Work out the finished part from the listing and answer in its coordinate system (mm). Face numbers are marked on the shaded views. A direction names the side the tool comes from. Round coordinates to 2 decimals unless told otherwise and drop trailing zeros. Write each loop counter-clockwise with the first axis right and the second up, starting at its lowest first coordinate (ties: lowest second). Pieces come first, ordered by that corner, then holes. Notation, with made-up numbers: M -4.5,-6.75 L -0.5,-6.75 A20 ccw -0.5,0.25 Z; hole C -4,74.25 d9. An arc over 180 degrees is marked long. Answer in a Markdown table with one row per item.
```python
from build123d import *

# Parameters (mm, degrees)
SKETCH_1_W          = 15
SKETCH_1_H          = 15
SKETCH_1_W_2        = 12
SKETCH_1_H_2        = 12
EXTRUDE_2_DEPTH     = 85
SKETCH_3_R          = 1.5
CUT_EXTRUDE_2_DEPTH = 10
SKETCH_4_R          = 1.5
CUT_EXTRUDE_3_DEPTH = 10
SKETCH_5_R          = 4
CUT_EXTRUDE_4_DEPTH = 10
SKETCH_6_R          = 4
CUT_EXTRUDE_5_DEPTH = 10
SKETCH_7_R          = 3
CUT_EXTRUDE_6_DEPTH = 10
SKETCH_8_R          = 1.5
CUT_EXTRUDE_7_DEPTH = 10
SKETCH_9_R          = 1.5
CUT_EXTRUDE_8_DEPTH = 10
SKETCH_10_R         = 4
CUT_EXTRUDE_9_DEPTH = 10


with BuildPart() as part:
    # ｽｹｯﾁ1 → ﾎﾞｽ - 押し出し2 (new body)
    with BuildSketch(Plane.XY):
        with Locations((0.489915859, 0.232626086)):
            Rectangle(SKETCH_1_W, SKETCH_1_H)
        with Locations((0.489915859, 0.232626086)):
            Rectangle(SKETCH_1_W_2, SKETCH_1_H_2, mode=Mode.SUBTRACT)
    extrude(amount=EXTRUDE_2_DEPTH)

    # ｽｹｯﾁ3 → ｶｯﾄ - 押し出し2 (cut)
    with BuildSketch(Plane(origin=(0, 7.732626086, 0), x_dir=(1, 0, 0), z_dir=(0, 1, 0))):
        with Locations((0.489915859, -77.5)):
            Circle(SKETCH_3_R)
    extrude(amount=-CUT_EXTRUDE_2_DEPTH, mode=Mode.SUBTRACT)

    # ｽｹｯﾁ4 → ｶｯﾄ - 押し出し3 (cut)
    with BuildSketch(Plane(origin=(7.989915859, 0, 0), x_dir=(0, 0, -1), z_dir=(1, 0, 0))):
        with Locations((-62.5, 0.232626086)):
            Circle(SKETCH_4_R)
    extrude(amount=-CUT_EXTRUDE_3_DEPTH, mode=Mode.SUBTRACT)

    # ｽｹｯﾁ5 → ｶｯﾄ - 押し出し4 (cut)
    with BuildSketch(Plane.XZ.offset(7.267373914)):
        with Locations((0.489915859, 77.5)):
            Circle(SKETCH_5_R)
    extrude(amount=-CUT_EXTRUDE_4_DEPTH, mode=Mode.SUBTRACT)

    # ｽｹｯﾁ6 → ｶｯﾄ - 押し出し5 (cut)
    with BuildSketch(Plane.ZY.offset(7.010084141)):
        with Locations((62.5, 0.232626086)):
            Circle(SKETCH_6_R)
    extrude(amount=-CUT_EXTRUDE_5_DEPTH, mode=Mode.SUBTRACT)

    # ｽｹｯﾁ7 → ｶｯﾄ - 押し出し6 (cut)
    with BuildSketch(Plane.ZY.offset(7.010084141)):
        with Locations((16, 0.232626086)):
            Circle(SKETCH_7_R)
    extrude(amount=-CUT_EXTRUDE_6_DEPTH, mode=Mode.SUBTRACT)

    # ｽｹｯﾁ8 → ｶｯﾄ - 押し出し7 (cut)
    with BuildSketch(Plane.ZY.offset(7.010084141)):
        with Locations((5, 0.232626086)):
            Circle(SKETCH_8_R)
    extrude(amount=-CUT_EXTRUDE_7_DEPTH, mode=Mode.SUBTRACT)

    # ｽｹｯﾁ9 → ｶｯﾄ - 押し出し8 (cut)
    with BuildSketch(Plane.ZY.offset(7.010084141)):
        with Locations((27, 0.232626086)):
            Circle(SKETCH_9_R)
    extrude(amount=-CUT_EXTRUDE_8_DEPTH, mode=Mode.SUBTRACT)

    # ｽｹｯﾁ10 → ｶｯﾄ - 押し出し9 (cut)
    with BuildSketch(Plane(origin=(7.989915859, 0, 0), x_dir=(0, 0, -1), z_dir=(1, 0, 0))):
        with Locations((-16, 0.232626086)):
            Circle(SKETCH_10_R)
        with Locations((-27, 0.232626086)):
            Circle(SKETCH_10_R)
    extrude(amount=-CUT_EXTRUDE_9_DEPTH, mode=Mode.SUBTRACT)


solid = part.part
```
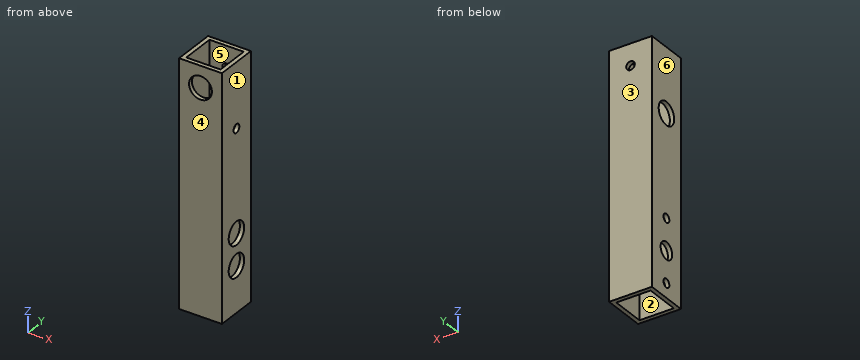
1. Given pin 1 (5 mm diameter, centred on x = 0.49, z = 77.5, fed in from +Y); pin 2 (5 mm diameter, centred on x = 0.49, z = 77.5, fed in from -Y); pin 3 (5 mm diameter, centred on y = 0.23, z = 62.5, fed in from -X), each flat-ended and moving along its own axis, determine where each tip first touches the part or whether it passes through.
Calculated:
| item | result |
|---|---|
| pin 1 | stops at y = 7.73 |
| pin 2 | stops at y = 6.23 |
| pin 3 | stops at x = 6.49 |
2. Determine the mould class of the marked faces 1, 2, 3 and 4 for opening direction Y: released by +Y, released by -Y, zero draft, split by the parting line, or undercut.
Calculated:
| item | result |
|---|---|
| face 1 | zero draft |
| face 2 | undercut |
| face 3 | released by +Y |
| face 4 | released by -Y |
3. The part is cut by section C-C (z = 62). Determine the outline of the cut face in (x, y), plus the area to 3 significant figures.
Calculated:
| item | result |
|---|---|
| outline | M -7.01,-7.27 L 7.99,-7.27 L 7.99,-1.18 L 6.49,-1.18 L 6.49,-5.77 L -5.51,-5.77 L -5.51,-3.74 L -7.01,-3.74 Z; M -7.01,4.2 L -5.51,4.2 L -5.51,6.23 L 6.49,6.23 L 6.49,1.65 L 7.99,1.65 L 7.99,7.73 L -7.01,7.73 Z |
| area | 64.9 mm² |
4. The part is cut by section B-B (y = -4.5). Determine the outline of the cut face in (x, z).
Calculated:
| item | result |
|---|---|
| outline | M -7.01,0 L -5.51,0 L -5.51,85 L -7.01,85 Z; M 6.49,0 L 7.99,0 L 7.99,85 L 6.49,85 Z |
5. Consider line 1 along Y through (x, z) = (5.75, 58); line 2 along X through (y, z) = (7.3, 77.5); line 3 along Y through (x, z) = (-6.25, 5). Determine where each line is inside the solid, lowest interval first. Write a range as from..to.
Calculated:
| item | result |
|---|---|
| line 1 | y = -7.27..-5.77, 6.23..7.73 |
| line 2 | x = -7.01..-1.01, 1.99..7.99 |
| line 3 | y = -7.27..-1.27, 1.73..7.73 |
6. The part is cut by section A-A (z = 39). Determine the outline of the cut face in (x, y), plus the area to 3 significant figures.
Calculated:
| item | result |
|---|---|
| outline | M -7.01,-7.27 L 7.99,-7.27 L 7.99,7.73 L -7.01,7.73 Z; hole M -5.51,-5.77 L 6.49,-5.77 L 6.49,6.23 L -5.51,6.23 Z |
| area | 81.0 mm² |
7. The part is cut by section D-D (x = -0.25). Determine the outline of the cut face in (y, z).
Calculated:
| item | result |
|---|---|
| outline | M -7.27,0 L -5.77,0 L -5.77,73.57 L -7.27,73.57 Z; M -7.27,81.43 L -5.77,81.43 L -5.77,85 L -7.27,85 Z; M 6.23,0 L 7.73,0 L 7.73,76.2 L 6.23,76.2 Z; M 6.23,78.8 L 7.73,78.8 L 7.73,85 L 6.23,85 Z |
8. A tool of negligible diameter and unlimited length cuts with its end or side. For the marked faces 5 and 6, from which of +Z, -Z, +X, -X, +Y, -Y can it reach the whole face along a straight path? Write none if from no direction.
Calculated:
| item | result |
|---|---|
| face 5 | +Z, -Z |
| face 6 | +Z, -Z, -X, +Y, -Y |
